Autodesk Inventor part; units mm, degrees
ref_plane "YZ Plane" through (0, 0, 0) normal (1, 0, 0) x (0, 1, 0)
ref_plane "XZ Plane" through (0, 0, 0) normal (0, 1, 0) x (-1, 0, 0)
ref_plane "XY Plane" through (0, 0, 0) normal (0, 0, 1) x (1, 0, 0)
sketch "草圖1" plane through (0, 0, 0) normal (0, 0, 1) x (1, 0, 0)
  line L0 (0, 0) -> (60, 0)
  line L1 (60, 0) -> (60, 10)
  line L2 (60, 10) -> (0, 10)
  line L3 (0, 10) -> (0, 0)
  circle A0 centre (40, 20) radius 10
  arc A1 (60, 20) -> (20, 20) centre (40, 20) ccw
  line L4 (20, 20) -> (20, 10)
  line L5 (60, 20) -> (60, 10)
  line L6 (20, 10) -> (0, 10)
  line L7 (0, 10) -> (0, 20)
  line L8 (0, 20) -> (20, 20)
  line L9 (20, 20) -> (20, 10)
  point P0 (40, 10)
  dimension "d0" = 60
  dimension "d1" = 10
  dimension "d2" = 20
  dimension "d3" = 40
  dimension "d4" = 10
  dimension "d5" = 20
  dimension "d10" = 20
  dimension "d11" = 10
extrude "擠出1" add sketch "草圖1" along normal blind 10 contours L7 L8 L4 L2 | L2 L4 A1 L5
extrude "擠出2" add sketch "草圖1" along normal blind 40 contours L3 L2 L1 L0
sketch "草圖2" plane through (0, 0, 40) normal (0, 0, 1) x (1, 0, 0)
  line L0 (0, 10) -> (0, 0)
  line L1 (0, 10) -> (20, 10)
  line L2 (20, 10) -> (20, 20)
  line L3 (10, 30) -> (0, 30)
  line L4 (0, 30) -> (0, 10)
  arc A0 (10, 30) -> (20, 20) centre (20, 30) ccw
extrude "擠出3" add sketch "草圖2" against normal blind 10
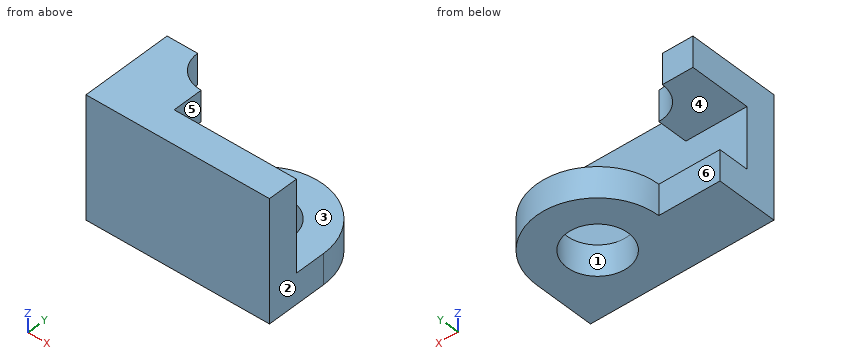
Geometry check sheet. Reference: the model listing, model coordinates, mm. Face numbers are marked on the shaded views. A direction names the side the tool comes from. Coordinates: 2 decimals unless noted, no trailing zeros. Write each loop counter-clockwise with the first axis right and the second up, starting at its lowest first coordinate (ties: lowest second). Pieces come first, ordered by that corner, then holes. Notation, with made-up numbers: (-30, -18.75) -> (1, -18.75) arc R27 ccw to (1, 6.25) -> close; hole circle Ø3 at (29.25, 83). An arc over 180 degrees is marked (long way). Use CSV: the item, a comma, the result in double quotes. Start each with the question number.
Item 1: Cross-section at B-B, the plane z = 6.5. Record the cut outline in (x, y), plus the area to 3 significant figures.
Item 2: Cross-section at A-A, the plane y = 13. Record the cut outline in (x, z), plus the area to 3 significant figures.
Item 3: Depth check by flat-ended pin: pin 1 Ø5 at (x, z) = (9.5, 4) entering from +Y; pin 2 Ø3 at (x, z) = (40.5, 17) entering from +Y; pin 3 Ø6 at (y, z) = (30, 10.5) entering from +X; pin 4 Ø3 at (x, y) = (18, 23) entering from -Z. Enter the tip coordinate at first touch or a pass-through.
Item 4: Thickness scan on line 1 (Z direction, x = 17, y = 12.5); line 2 (Y direction, x = 43, z = 35). Record the ranges inside material, lowest first.
Item 5: Cross-section at D-D, the plane z = 32. Record the cut outline in (x, y).
Item 6: Set-up check for the marked faces 4, 5 and 6: record each of +Z, -Z, +X, -X, +Y, -Y from which the full face is reachable in a straight line by a thin tool's end or side.
Item 7: Cross-section at C-C, the plane x = 24. Record the cut outline in (y, z).
Item 8: Mould release check, pull along X, two halves, no side actions. Record for the marked faces 1, 2 and 3: released by +X, released by -X, zero draft, split by the parting line, or undercut.
Answers:
1,outline,"(0, 0) -> (60, 0) -> (60, 20) arc R20 ccw to (20, 20) -> (0, 20) -> close; hole circle Ø20 at (40, 20)"
1,area,"1,510 mm^2"
2,outline,"(0, 0) -> (32.86, 0) -> (32.86, 10) -> (0, 10) -> close; (0, 30) -> (20, 30) -> (20, 40) -> (0, 40) -> close; (47.14, 0) -> (60, 0) -> (60, 10) -> (47.14, 10) -> close"
2,area,"657 mm^2"
3,pin 1,"y = 20"
3,pin 2,"y = 10"
3,pin 3,"x = 58.72"
3,pin 4,"through"
4,line 1,"0 to 10, 30 to 40"
4,line 2,"0 to 10"
5,outline,"(0, 0) -> (60, 0) -> (60, 10) -> (20, 10) -> (20, 20) arc R10 cw to (10, 30) -> (0, 30) -> close"
6,face 4,"+X, -X, +Y"
6,face 5,"+Z, +X, +Y"
6,face 6,"-Z, -X, +Y"
7,outline,"(0, 0) -> (32, 0) -> (32, 10) -> (10, 10) -> (10, 40) -> (0, 40) -> close"
8,face 1,"undercut"
8,face 2,"released by +X"
8,face 3,"zero draft"
